from build123d import *

# Parameters (mm, degrees)
SKETCH1_R           = 1.65
BOSS_EXTRUDE1_DEPTH = 3


with BuildPart() as part:
    # Sketch1 → Boss-Extrude1 (new body)
    with BuildSketch(Plane.XY):
        Polygon((0, -26), (44.5, -26), (44.5, 2), (64.5, 2), (64.5, -26), (140, -26), (140, 22), (140, 66), (140, 114), (64.5, 114), (64.5, 86), (44.5, 86), (44.5, 114), (0, 114), (0, 66), (10, 60), (10, 28), (0, 22), align=None)
        with Locations((10, 22)):
            Circle(SKETCH1_R, mode=Mode.SUBTRACT)
        with Locations(Location((130, 66, 0), (0, 0, 180))):
            Circle(SKETCH1_R, mode=Mode.SUBTRACT)
        with Locations((130, 22)):
            Circle(SKETCH1_R, mode=Mode.SUBTRACT)
        with Locations(Location((10, 66, 0), (0, 0, 180))):
            Circle(SKETCH1_R, mode=Mode.SUBTRACT)
    extrude(amount=BOSS_EXTRUDE1_DEPTH)


solid = part.part
Model file for the job. Use its own axes, mm. A direction names the side the tool comes from. Coordinates: 2 decimals unless noted, no trailing zeros. Write each loop counter-clockwise with the first axis right and the second up, starting at its lowest first coordinate (ties: lowest second). Pieces come first, ordered by that corner, then holes. Notation, with made-up numbers: (-38.75, 60) -> (18.25, 60) arc R28 cw to (18.25, 91) -> close; hole circle Ø3 at (-7.5, -16). An arc over 180 degrees is marked (long way). One line per item, written item: value. Start each with the question number.
1) Flat gauge pins, fed straight in: pin 1 Ø0.9 at (x, z) = (50.5, 1.5) entering from +Y; pin 2 Ø1.5 at (x, z) = (52, 2) entering from -Y; pin 3 Ø2 at (x, y) = (10, 66) entering from +Z; pin 4 Ø1.5 at (y, z) = (46, 1) entering from -X. Where does each tip first touch, or does it go through?
2) Which spindle directions (+Z, -Z, +X, -X, +Y, -Y) get a long thin tool onto all of the face, cutting with end or side? Do faces 5 (the face through (10, 44, 1)), 6 (the face through (55, 86, 1)), 7 (the face through (54, 2, 1)), 8 (the face through (0, 90, 1)). Say none if no direction does.
3) Slice it at B-B on z = 1. Write the cut outline in (x, y), then the cut area to 3 significant figures.
4) Pull direction X, two halves, no side cores. Call faces 1 (the face through (10.89, 23.39, 1.48)), 2 (the face through (140, 43, 1)), 3 (the face through (5, 63, 1)), 4 (the face through (128.476, 66.632, 1.479)): +X half, -X half, draft (parallel to the pull), parting line (faces both ways), or undercut.
5) Slice it at A-A on y = -14. Write the cut outline in (x, z), then the cut area to 3 significant figures.
6) Slice it at D-D on x = 62.5. Write the cut outline in (y, z).
7) Slice it at C-C on x = 130. Write the cut outline in (y, z), then the cut area to 3 significant figures.
8) Probe probe 1 along X at (y, z) = (66, 2.1); probe 2 along Y at (x, z) = (130, 1.3); probe 3 along X at (y, z) = (-11, 0.5). List the from-to ranges inside material, lowest first.
Answers follow:
1. pin 1: y = 86
1. pin 2: y = 2
1. pin 3: through
1. pin 4: x = 10
2. face 5: +Z, -Z, -X
2. face 6: +Z, -Z, +Y
2. face 7: +Z, -Z, -Y
2. face 8: +Z, -Z, -X, +Y, -Y
3. outline: (0, -26) -> (44.5, -26) -> (44.5, 2) -> (64.5, 2) -> (64.5, -26) -> (140, -26) -> (140, 114) -> (64.5, 114) -> (64.5, 86) -> (44.5, 86) -> (44.5, 114) -> (0, 114) -> (0, 66) -> (10, 60) -> (10, 28) -> (0, 22) -> close; hole circle Ø3.3 at (10, 22); hole circle Ø3.3 at (10, 66); hole circle Ø3.3 at (130, 22); hole circle Ø3.3 at (130, 66)
3. area: 18,100 mm2
4. face 1: undercut
4. face 2: +X half
4. face 3: -X half
4. face 4: undercut
5. outline: (0, 0) -> (44.5, 0) -> (44.5, 3) -> (0, 3) -> close; (64.5, 0) -> (140, 0) -> (140, 3) -> (64.5, 3) -> close
5. area: 360 mm2
6. outline: (2, 0) -> (86, 0) -> (86, 3) -> (2, 3) -> close
7. outline: (-26, 0) -> (20.35, 0) -> (20.35, 3) -> (-26, 3) -> close; (23.65, 0) -> (64.35, 0) -> (64.35, 3) -> (23.65, 3) -> close; (67.65, 0) -> (114, 0) -> (114, 3) -> (67.65, 3) -> close
7. area: 400 mm2
8. probe 1: 0 to 8.35, 11.65 to 128.35, 131.65 to 140
8. probe 2: -26 to 20.35, 23.65 to 64.35, 67.65 to 114
8. probe 3: 0 to 44.5, 64.5 to 140
